```python
from build123d import *

# Parameters (mm, degrees)
ESBO_O1_R                = 11
RESSALTO_EXTRUS_O1_DEPTH = 13
ESBO_O2_R                = 7.5
RESSALTO_EXTRUS_O2_DEPTH = 4
ESBO_O3_R                = 5.5
RESSALTO_EXTRUS_O3_DEPTH = 13
ESBO_O4_R                = 3
RESSALTO_EXTRUS_O4_DEPTH = 3
ESBO_O5_R                = 4.5
RESSALTO_EXTRUS_O5_DEPTH = 32
CHANFRO1_SIZE            = 1
CHANFRO2_SIZE            = 1
ESBO_O6_R                = 1.5


with BuildPart() as part:
    # Esboço1 → Ressalto-extrusão1 (new body)
    with BuildSketch(Plane.XY):
        with Locations(Location((0, 0, 0), (0, 0, 180))):
            Circle(ESBO_O1_R)
    extrude(amount=RESSALTO_EXTRUS_O1_DEPTH)

    # Esboço2 → Ressalto-extrusão2 (add)
    with BuildSketch(Plane.XY.offset(13)):
        Circle(ESBO_O2_R)
    extrude(amount=RESSALTO_EXTRUS_O2_DEPTH)

    # Esboço3 → Ressalto-extrusão3 (add)
    with BuildSketch(Plane.XY.offset(17)):
        with Locations(Location((0, 0, 0), (0, 0, 180))):
            Circle(ESBO_O3_R)
    extrude(amount=RESSALTO_EXTRUS_O3_DEPTH)

    # Esboço4 → Ressalto-extrusão4 (add)
    with BuildSketch(Plane.XY.offset(30)):
        Circle(ESBO_O4_R)
    extrude(amount=RESSALTO_EXTRUS_O4_DEPTH)

    # Esboço5 → Ressalto-extrusão5 (add)
    with BuildSketch(Plane.XY.offset(33)):
        Circle(ESBO_O5_R)
    extrude(amount=RESSALTO_EXTRUS_O5_DEPTH)

    # Chanfro1
    chanfro1_edges = [part.edges().sort_by_distance(p)[0] for p in [
        (11, 0, 0),
    ]]
    chamfer(chanfro1_edges, length=CHANFRO1_SIZE)

    # Chanfro2
    chanfro2_edges = [part.edges().sort_by_distance(p)[0] for p in [
        (5.5, 0, 30),
        (-4.5, 0, 65),
        (11, 0, 13),
    ]]
    chamfer(chanfro2_edges, length=CHANFRO2_SIZE)

    # Varredura de corte1: sweep along a path in Esboço7
    with BuildLine(Plane.XY.offset(23.5)) as varredura_de_corte1_path:
        CenterArc((0, 0), 5.5, 0, 360)
    # Esboço6 → Varredura de corte1 (sweep, cut)
    with BuildSketch(Plane(origin=(0, 0, 0), x_dir=(1, 0, 0), z_dir=(0, 1, 0))):
        with Locations((-5.5, -23.5)):
            Circle(ESBO_O6_R)
    sweep(path=varredura_de_corte1_path.line, mode=Mode.SUBTRACT)


solid = part.part
```
Build history of the part. All positions in model axes, mm. A direction names the side the tool comes from. Give positions to 0.01 mm unless a question says otherwise; leave off trailing zeros. Order: outer loops, then holes, each group sorted by start corner. A loop starts at its lowest first (then second) coordinate and runs counter-clockwise, first axis right, second up. Notation, with made-up numbers: M 11,35.5 L 19,35.5 A15 cw 19,51.5 Z; hole C 77,2.25 d11. An arc over 180 degrees is marked long. Write item = value, one per line. Start each with the question number.
(1) Slice it at D-D on z = 10. Write the cut outline in (x, y), plus the area to 3 significant figures.
(2) Slice it at C-C on z = 57. Write the cut outline in (x, y), plus the area to 3 significant figures.
(3) Which spindle directions (+Z, -Z, +X, -X, +Y, -Y) get a long thin tool onto all of the face, cutting with end or side? Do faces 1 (the flat face through (0, 0, 65)), 2 (the cylindrical face through (-0.59, 4.46, 48.28)), 3 (the flat face through (-1, 3, 30)). Say none if no direction does.
(4) Probe L1, parallel to Z at x = 9.75, y = 0; L2, parallel to Z at x = 4.75, y = -4.5; L3, parallel to Z at x = -4.25, y = -1.75. List the from-to ranges inside material, lowest first. Write a range as [from, to].
(5) Two-plate mould, pull along Z, no slides. Class faces 4 (the flat face through (1, -3, 33)), 5 (the flat face through (-4, 4, 17)), 6 (the cylindrical face through (2.38, 10.74, 6.42)): released by +Z, released by -Z, zero draft, split by the parting line, or undercut.
(6) Pin check, flat tips, straight feed: pin 1 Ø4 at (x, z) = (-4, 36.5) entering from -Y; pin 2 Ø3 at (x, y) = (7.5, 7.5) entering from -Z; pin 3 Ø1 at (x, y) = (-8, -9) entering from +Z; pin 4 Ø1.5 at (x, z) = (0.5, 28) entering from -Y. Stop position of each tip, or through.
Responses:
q1.outline = C 0,0 d22
q1.area = 380 mm2
q2.outline = C 0,0 d9
q2.area = 63.6 mm2
q3.face_1 = +Z, +X, -X, +Y, -Y
q3.face_2 = +Z
q3.face_3 = none
q4.L1 = [0, 13]
q4.L2 = [0, 17]
q4.L3 = [0, 22.3], [24.7, 29.9]
q5.face_4 = undercut
q5.face_5 = released by +Z
q5.face_6 = zero draft
q6.pin_1 = -4.03
q6.pin_2 = 0
q6.pin_3 = through
q6.pin_4 = -5.5
